```python
from build123d import *

# Parameters (mm, degrees)
F0_R      = 63.5
F1_DEPTH  = 25.4
F3_DEPTH  = 17.4625
F4_R      = 6.35
F5_DEPTH  = 19.05
F6_R      = 21.59
F7_DEPTH  = 25.4
F8_R      = 32.54375
F8_R_2    = 21.59
F9_DEPTH  = 12.7
F11_DEPTH = 9.525


with BuildPart() as f1:
    # F0 (on Top) → F1 (new body)
    with BuildSketch(Plane.XY):
        Circle(F0_R)
    extrude(amount=F1_DEPTH)

    # F2 (on face) → F3 (cut)
    with BuildSketch(Plane.XY.offset(25.4)):
        with BuildLine():
            ThreePointArc((50.8, -38.1), (63.5, 0), (50.8, 38.1))
            Line((50.8, 38.1), (50.8, -38.1))
        make_face()
    extrude(amount=-F3_DEPTH, mode=Mode.SUBTRACT)

    # F4 (on face) → F5 (cut)
    with BuildSketch(Plane.XY.offset(25.4)):
        with Locations((0, 44.45)):
            Circle(F4_R)
        with Locations((-44.45, 0)):
            Circle(F4_R)
        with Locations((0, -44.45)):
            Circle(F4_R)
    extrude(amount=-F5_DEPTH, mode=Mode.SUBTRACT)

    # F6 (on face) → F7 (cut, through all)
    with BuildSketch(Plane.XY.offset(25.4)):
        Circle(F6_R)
    extrude(amount=-F7_DEPTH, mode=Mode.SUBTRACT)

    # F8 (on face) → F9 (join)
    with BuildSketch(Plane(origin=(0, 0, 0), x_dir=(1, 0, 0), z_dir=(0, 0, -1))):
        Circle(F8_R)
        Circle(F8_R_2, mode=Mode.SUBTRACT)
    extrude(amount=F9_DEPTH)

    # F10 (on face) → F11 (join)
    with BuildSketch(Plane.YZ.offset(50.8)):
        Polygon((-31.75, 7.9375), (0, 7.9375), (31.75, 7.9375), (31.75, 42.8625), (0, 42.8625), (-31.75, 42.8625), align=None)
    extrude(amount=F11_DEPTH)


solid = f1.part
```
Can you work these out from the model? Positions are in its coordinate system, mm. A direction names the side the tool comes from. Coordinates: 2 decimals unless noted, no trailing zeros. Order: outer loops, then holes, each group sorted by start corner. A loop starts at its lowest first (then second) coordinate and runs counter-clockwise, first axis right, second up.
1. I need wall thicknesses on line 1 (Y direction, x = 0, z = 8); line 2 (X direction, y = 0, z = -10); line 3 (X direction, y = -4.5, z = 24.5) (3 decimals). Which ranges of each line are inside material? Lowest first, please.
2. If we section it at A-A (x = 0): Please give me the cut outline in (y, z), then the cut area to 3 significant figures.
3. Thinking about a two-plate mould opening in X: for faces 4 (the face through (-25.826, 19.802, -6.261)), 5 (the face through (-38.393, 1.907, 16.008)), 6 (the face through (50.8, 0, 34)), 7 (the face through (-15, 29.1, 0)), which applies, +X half, -X half, draft (parallel to the pull), parting line (faces both ways), or undercut?
4. For faces 1 (the face through (-20, 15, 25.4)), 2 (the face through (-0.827, 50.746, 16.008)), 3 (the face through (52, -34, 7.938)), which set-ups out of +Z, -Z, +X, -X, +Y, -Y let a thin tool reach every point of the face, with its end or its side?
5. If we section it at D-D (x = -44.45): Please give me the cut outline in (y, z), then the cut area to 3 significant figures.
6. I'm going to push flat-ended pins straight in: pin 1 (4 mm diameter, centred on y = 36.5, z = 9, fed in from -X); pin 2 (10.5 mm diameter, centred on y = 5, z = 29.5, fed in from +X) (3 decimals); pin 3 (10.5 mm diameter, centred on x = 57, z = 26.5, fed in from -Y). Where does each tip first touch, or does it pass through?
7. If we section it at C-C (z = 11): Please give me the cut outline in (x, y) (3 decimals).
Entries:
1. line 1: y = -63.5 to -50.8, -38.1 to -21.59, 21.59 to 38.1, 50.8 to 63.5
1. line 2: x = -32.54 to -21.59, 21.59 to 32.54
1. line 3: x = -63.34 to -48.93, -39.97 to -21.116, 21.116 to 60.325
2. outline: (-63.5, 0) - (-32.54, 0) - (-32.54, -12.7) - (-21.59, -12.7) - (-21.59, 25.4) - (-38.1, 25.4) - (-38.1, 6.35) - (-50.8, 6.35) - (-50.8, 25.4) - (-63.5, 25.4) - close; (21.59, -12.7) - (32.54, -12.7) - (32.54, 0) - (63.5, 0) - (63.5, 25.4) - (50.8, 25.4) - (50.8, 6.35) - (38.1, 6.35) - (38.1, 25.4) - (21.59, 25.4) - close
2. area: 1,920 mm2
3. face 4: parting line
3. face 5: undercut
3. face 6: -X half
3. face 7: draft
4. face 1: +Z, -X, +Y, -Y
4. face 2: +Z
4. face 3: +Z, +X, -Y
5. outline: (-45.35, 0) - (45.35, 0) - (45.35, 25.4) - (6.35, 25.4) - (6.35, 6.35) - (-6.35, 6.35) - (-6.35, 25.4) - (-45.35, 25.4) - close
5. area: 2,060 mm2
6. pin 1: stops at x = -53.31
6. pin 2: stops at x = 60.325
6. pin 3: stops at y = -31.75
7. outline: (50.8, -38.1) - (50.8, -31.75) - (60.325, -31.75) - (60.325, 31.75) - (50.8, 31.75) - (50.8, 38.1) arc R63.5 ccw (long way) to start; hole circle Ø12.7 at (-44.45, 0); hole circle Ø43.18 at (0, 0); hole circle Ø12.7 at (0, -44.45); hole circle Ø12.7 at (0, 44.45)
